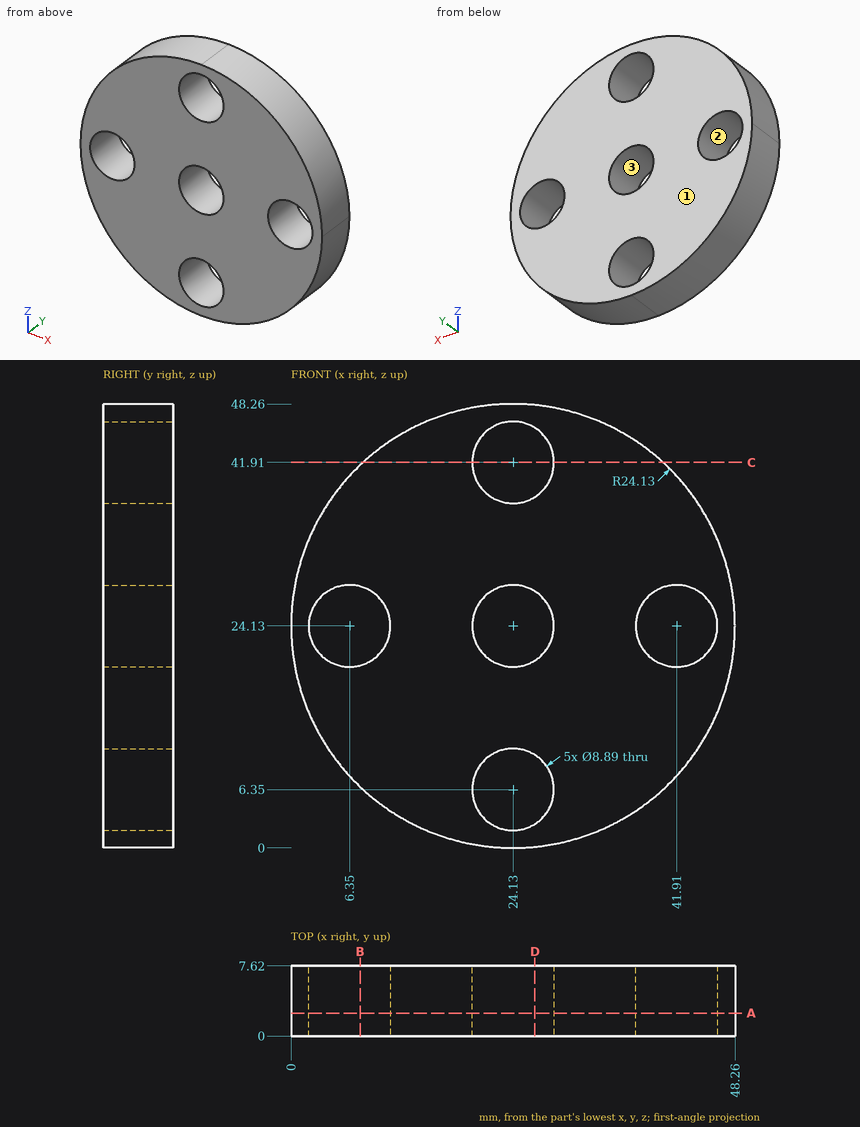
Check sheet for the drawn part. Datum: minimum x, y, z corner. Units: mm. Coordinates: 2 decimals unless noted, no trailing zeros. Order: outer loops, then holes, each group sorted by start corner. A loop starts at its lowest first (then second) coordinate and runs counter-clockwise, first axis right, second up. Notation, with made-up numbers: M 72,28.5 L 83,28.5 A13 cw 83,34.5 Z; hole C 86.5,59 d3. An arc over 180 degrees is marked long. One line per question, with ' | ' between items. Start each with the question number.
Item 1: Sectioned sample at D-D on x = 26.5. Record the cut outline in (y, z).
Item 2: Mould release check, pull along X, two halves, no side actions. Record for the marked faces 1, 2 and 3: pulls with the +X half, pulls with the -X half, needs draft (parallel to the pull), parting line crosses it, or undercut.
Item 3: Sectioned sample at A-A on y = 2.5. Record the cut outline in (x, z) (3 decimals).
Item 4: Sectioned sample at C-C on z = 41.91. Record the cut outline in (x, y) (3 decimals).
Item 5: Gauge pin test, flat ends, axial feed: P1, Ø7, axis at x = 24.13, z = 6.35, coming from the +Y side; P2, Ø2, axis at y = 5, z = 34, coming from the -X side; P3, Ø4, axis at y = 1, z = 5.5, coming from the -X side. Record the tip position at first contact, or that the pin passes through.
Item 6: Material ranges on line 1 (X direction, y = 6.5, z = 24); line 2 (Z direction, x = 24.13, y = 2) (3 decimals); line 3 (Z direction, x = 27, y = 3.5), recorded low to high.
Item 7: Sectioned sample at B-B on x = 7.5. Record the cut outline in (y, z), and give its area (3 significant figures).
Answer below:
1) outline: M 0,0.12 L 7.62,0.12 L 7.62,2.59 L 0,2.59 Z; M 0,10.11 L 7.62,10.11 L 7.62,20.37 L 0,20.37 Z; M 0,27.89 L 7.62,27.89 L 7.62,38.15 L 0,38.15 Z; M 0,45.67 L 7.62,45.67 L 7.62,48.14 L 0,48.14 Z
2) face 1: needs draft | face 2: undercut | face 3: undercut
3) outline: C 24.13,24.13 d48.26; hole C 6.35,24.13 d8.89; hole C 24.13,6.35 d8.89; hole C 24.13,24.13 d8.89; hole C 24.13,41.91 d8.89; hole C 41.91,24.13 d8.89
4) outline: M 7.817,0 L 19.685,0 L 19.685,7.62 L 7.817,7.62 Z; M 28.575,0 L 40.443,0 L 40.443,7.62 L 28.575,7.62 Z
5) P1: passes through | P2: stops at x = 1.69 | P3: stops at x = 6.65
6) line 1: x = 0 to 1.91, 10.79 to 19.69, 28.57 to 37.47, 46.35 to 48.26 | line 2: z = 0 to 1.905, 10.795 to 19.685, 28.575 to 37.465, 46.355 to 48.26 | line 3: z = 0.17 to 2.96, 9.74 to 20.74, 27.52 to 38.52, 45.3 to 48.09
7) outline: M 0,6.65 L 7.62,6.65 L 7.62,19.84 L 0,19.84 Z; M 0,28.42 L 7.62,28.42 L 7.62,41.61 L 0,41.61 Z | area: 201 mm^2
